Input: part model. Units: mm. Frame: model coordinates. Face numbers are marked on the shaded views. A direction names the side the tool comes from. Round coordinates to 2 decimals unless told otherwise and drop trailing zeros. Loops run counter-clockwise (first coordinate to the right, second up) from the corner with the lowest first, then second, coordinate; pieces in that order, holes last. Notation, with made-up numbers: (14, 14) -> (49, 14) arc R28 cw to (49, 37) -> close; hole circle Ø3 at (11, 87.5). An arc over 180 degrees is marked (long way). Answer in a Markdown table with one row per item. Add a question column.
Q1. Mould query, pull axis X, two halves, no side actions, for the marked faces 3, 4 and 5. Classes: pulls with the +X half, pulls with the -X half, needs draft (parallel to the pull), parting line crosses it, or undercut.
Q2. Pin query (flat end, axial travel): pin 1 (5 mm diameter, centred on x = 0, z = -2, fed in from +Y). Return the tip coordinate at first contact, or that it passes through.
Q3. Section B-B, the plane z = 11.25. Output: boundary loops of the cut face in (x, y).
Q4. Section C-C, the plane x = 0.75. Output: boundary loops of the cut face in (y, z), and give its area (3 significant figures).
Q5. Section A-A, the plane y = 6. Output: boundary loops of the cut face in (x, z).
Q6. Ray query, L1, parallel to Z at x = 2.5, y = 4.25; L2, parallel to X at y = 3.5, z = -10; L3, parallel to Y at x = -3.25, z = -8.75. Return the intervals inside material, ascending. Write a range as from..to.
Q7. Reachability of the marked faces 1 and 2 from +Z, -Z, +X, -X, +Y, -Y: full face, straight path, thin tool, end or side. Return the list, or none.
Autodesk Inventor part; units mm, degrees
ref_plane "YZ Plane" through (0, 0, 0) normal (1, 0, 0) x (0, 1, 0)
ref_plane "XZ Plane" through (0, 0, 0) normal (0, 1, 0) x (-1, 0, 0)
ref_plane "XY Plane" through (0, 0, 0) normal (0, 0, 1) x (1, 0, 0)
sketch "Sketch1" plane through (0, 0, 0) normal (0, 1, 0) x (-1, 0, 0)
  line L0 (6.0929, 13.5835) -> (-6.0929, 13.5835)
  line L1 (-6.0929, 13.5835) -> (-6.0929, -13.5835)
  line L2 (-6.0929, -13.5835) -> (6.0929, -13.5835)
  line L3 (6.0929, -13.5835) -> (6.0929, 13.5835)
  line L4 (6.0929, 13.5835) -> (-6.0929, -13.5835) construction
  line L5 (-6.0929, 13.5835) -> (6.0929, -13.5835) construction
  point P0 (0, 0)
extrude "Extrusion1" add sketch "Sketch1" along normal blind 10
shell "Shell1" thickness 1 removed faces 1 at (2.031, 10, -4.5278)
equation "\"BendRadius\" = Thickness"
equation "\"BendReliefWidth\" = Thickness"
equation "\"BendReliefDepth\" = 0.5 * Thickness"
equation "\"CornerReliefSize\" = 4 * Thickness"
equation "\"MinimumRemnant\" = 2 * Thickness"
equation "\"TransitionRadius\" = BendRadius"
equation "\"JacobiRadiusSize\" = BendRadius"
equation "\"GapSize\" = Thickness"
properties part number "Stress analysis" material "Aluminum 6061-AHC"
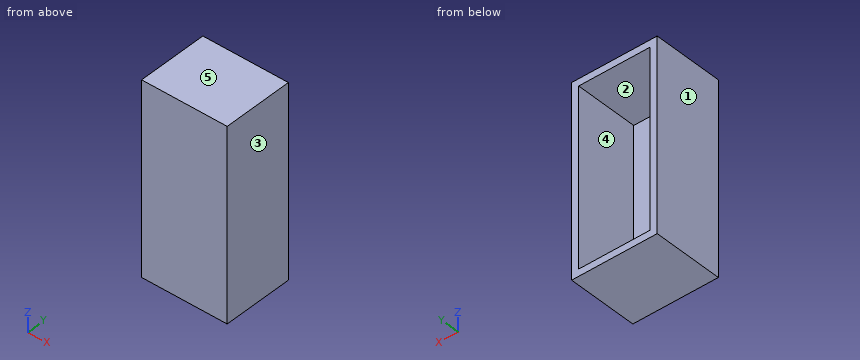
Answer block:
| question | item | result |
|---|---|---|
| 1 | face 3 | pulls with the +X half |
| 1 | face 4 | undercut |
| 1 | face 5 | needs draft |
| 2 | pin 1 | y = 1 |
| 3 | outline | (-6.09, 0) -> (6.09, 0) -> (6.09, 10) -> (5.09, 10) -> (5.09, 1) -> (-5.09, 1) -> (-5.09, 10) -> (-6.09, 10) -> close |
| 4 | outline | (0, -13.58) -> (10, -13.58) -> (10, -12.58) -> (1, -12.58) -> (1, 12.58) -> (10, 12.58) -> (10, 13.58) -> (0, 13.58) -> close |
| 4 | area | 45.2 mm^2 |
| 5 | outline | (-6.09, -13.58) -> (6.09, -13.58) -> (6.09, 13.58) -> (-6.09, 13.58) -> close; hole (-5.09, -12.58) -> (5.09, -12.58) -> (5.09, 12.58) -> (-5.09, 12.58) -> close |
| 6 | L1 | -13.58..-12.58, 12.58..13.58 |
| 6 | L2 | -6.09..-5.09, 5.09..6.09 |
| 6 | L3 | 0..1 |
| 7 | face 1 | +Z, -Z, -X, +Y, -Y |
| 7 | face 2 | +Y |
